```python
from build123d import *

# Parameters (mm, degrees)
SKETCH2_W                = 12
SKETCH2_H                = 90
BOSS_EXTRUDE1_DEPTH      = 10
FILLET1_R                = 5
CUT_EXTRUDE1_DEPTH       = 3
CUT_EXTRUDE2_START       = 7
SKETCH3_2_W              = 12
SKETCH3_2_H              = 9
CUT_EXTRUDE2_DEPTH       = 3
CUT_EXTRUDE4_START       = -4
CUT_EXTRUDE4_DEPTH       = 51.486557197
SKETCH7_R                = 1.5
CUT_EXTRUDE5_DEPTH       = 46.934736311
BOSS_EXTRUDE2_DEPTH      = 7
BOSS_EXTRUDE2_DEPTH_BACK = 7
SKETCH9_W                = 15
SKETCH9_H                = 60
FILLET3_R                = 7


with BuildPart() as part:
    # Sketch2 → Boss-Extrude1 (new body)
    with BuildSketch(Plane.XY):
        Rectangle(SKETCH2_W, SKETCH2_H)
    extrude(amount=BOSS_EXTRUDE1_DEPTH)

    # Fillet1
    fillet1_edges = [part.edges().sort_by_distance(p)[0] for p in [
        (-6, 0, 0),
        (6, 0, 0),
        (6, 0, 10),
        (-6, 0, 10),
    ]]
    fillet(fillet1_edges, radius=FILLET1_R - 0.0001)  # a hair under: the kernel refuses the full size

    # Sketch3 → Cut-Extrude1 (cut)
    with BuildSketch(Plane.XY):
        with BuildLine():
            Line((-6, -36), (-4.5, -40.5))
            ThreePointArc((-4.5, -40.5), (0, -45), (4.5, -40.5))
            Line((4.5, -40.5), (6, -36))
            Line((6, -36), (-6, -36))
        make_face()
        with BuildLine():
            Line((-3.9e-08, -45), (6, -45))
            Line((6, -45), (6, -36))
            Line((6, -36), (4.5, -40.5))
            ThreePointArc((4.5, -40.5), (3.181980501, -43.681980529), (-3.9e-08, -45))
        make_face()
        with BuildLine():
            Line((-6, -45), (-3.9e-08, -45))
            ThreePointArc((-3.9e-08, -45), (-3.181980529, -43.681980501), (-4.5, -40.5))
            Line((-4.5, -40.5), (-6, -36))
            Line((-6, -36), (-6, -45))
        make_face()
    cut_extrude1 = extrude(amount=CUT_EXTRUDE1_DEPTH, mode=Mode.SUBTRACT)

    # Sketch3<2> → Cut-Extrude2 (cut)
    with BuildSketch(Plane.XY.offset(CUT_EXTRUDE2_START)):
        with Locations((0, -40.5)):
            Rectangle(SKETCH3_2_W, SKETCH3_2_H)
    cut_extrude2 = extrude(amount=CUT_EXTRUDE2_DEPTH, mode=Mode.SUBTRACT)

    # Mirror1: Cut-Extrude1, Cut-Extrude2 across plane
    add(cut_extrude1.mirror(Plane.ZX), mode=Mode.SUBTRACT)
    add(cut_extrude2.mirror(Plane.ZX), mode=Mode.SUBTRACT)

    # Sketch3<4> → Cut-Extrude4 (cut)
    with BuildSketch(Plane.XY.offset(CUT_EXTRUDE4_START)):
        with BuildLine():
            Line((-3.9e-08, -45), (6, -45))
            Line((6, -45), (6, -36))
            Line((6, -36), (4.5, -40.5))
            ThreePointArc((4.5, -40.5), (3.181980501, -43.681980529), (-3.9e-08, -45))
        make_face()
        with BuildLine():
            Line((-6, -45), (-3.9e-08, -45))
            ThreePointArc((-3.9e-08, -45), (-3.181980529, -43.681980501), (-4.5, -40.5))
            Line((-4.5, -40.5), (-6, -36))
            Line((-6, -36), (-6, -45))
        make_face()
    cut_extrude4 = extrude(amount=CUT_EXTRUDE4_DEPTH, mode=Mode.SUBTRACT)

    # Sketch7 → Cut-Extrude5 (cut, through all)
    with BuildSketch(Plane(origin=(0, 0, 3), x_dir=(-1, 0, 0), z_dir=(0, 0, -1))):
        with Locations((0, -40.5)):
            Circle(SKETCH7_R)
    cut_extrude5 = extrude(amount=-CUT_EXTRUDE5_DEPTH, mode=Mode.SUBTRACT)

    # Mirror3: Cut-Extrude5 across plane
    add(cut_extrude5.mirror(Plane.ZX), mode=Mode.SUBTRACT)

    # Mirror4: Cut-Extrude4 across plane
    add(cut_extrude4.mirror(Plane.ZX), mode=Mode.SUBTRACT)

    # Sketch9 → Boss-Extrude2 (add, two sides: drawn at the far end of the back side and taken through both)
    with BuildSketch(Plane.XY.offset(5).offset(-BOSS_EXTRUDE2_DEPTH_BACK)):
        Rectangle(SKETCH9_W, SKETCH9_H)
    extrude(amount=BOSS_EXTRUDE2_DEPTH + BOSS_EXTRUDE2_DEPTH_BACK)

    # Fillet3
    fillet3_edges = [part.edges().sort_by_distance(p)[0] for p in [
        (-7.5, 0, 12),
        (7.5, 0, 12),
        (7.5, 0, -2),
        (-7.5, 0, -2),
    ]]
    fillet(fillet3_edges, radius=FILLET3_R - 0.0001)  # a hair under: the kernel refuses the full size


solid = part.part
```
Can you work these out from the model? Positions are in its coordinate system, mm. A direction names the side the tool comes from. Coordinates: 2 decimals unless noted, no trailing zeros. Loops run counter-clockwise (first coordinate to the right, second up) from the corner with the lowest first, then second, coordinate; pieces in that order, holes last.
Item 1: Please list where these lines run through material, in increasing order: L1, parallel to Y at x = 0, z = 4.2; L2, parallel to X at y = 40.5, z = 4.9; L3, parallel to Y at x = -1, z = 6.5.
Answers below:
L1: y = -45 to -42, -39 to 39, 42 to 45
L2: x = -4.5 to -1.5, 1.5 to 4.5
L3: y = -44.89 to -41.62, -39.38 to 39.38, 41.62 to 44.89
Item 2: If we mould it in two halves opening along Y, with no side actions, what happens to faces 1 (the face through (0, 33, 10)), 2 (the face through (5.26, -38.22, 4.97)), 3 (the face through (0, 36, 8)), 4 (the face through (0, -42, 5))? For each: released by +Y, released by -Y, zero draft, split by the parting line, or undercut.
Answers below:
face 1: zero draft
face 2: released by -Y
face 3: released by +Y
face 4: undercut
Item 3: I'm going to push flat-ended pins straight in: pin 1 (2 mm diameter, centred on x = 0.5, y = 32, fed in from -Z); pin 2 (0.9 mm diameter, centred on x = 2.5, z = 2, fed in from +Y); pin 3 (7 mm diameter, centred on x = 0.5, y = 42.5, fed in from +Z); pin 4 (3 mm diameter, centred on y = -1.5, z = 5.5, fed in from -X). Where does each tip first touch, or does it pass through?
Answers below:
pin 1: stops at z = 0
pin 2: stops at y = 36
pin 3: stops at z = 7
pin 4: stops at x = -7.5
Item 4: Suppose I cut it at B-B (z = 8.25). Please give me the cut outline in (x, y).
Answers below:
outline: (-6.7, -30) - (-4.8, -30) - (-4.8, -36) - (4.8, -36) - (4.8, -30) - (6.7, -30) - (6.7, 30) - (4.8, 30) - (4.8, 36) - (-4.8, 36) - (-4.8, 30) - (-6.7, 30) - close
Item 5: Suppose I cut it at C-C (x = 2.5). Please give me the cut outline in (y, z).
Answers below:
outline: (-44.24, 3) - (-36, 3) - (-36, 0.23) - (-30, 0.23) - (-30, -1.71) - (30, -1.71) - (30, 0.23) - (36, 0.23) - (36, 3) - (44.24, 3) - (44.24, 7) - (36, 7) - (36, 9.77) - (30, 9.77) - (30, 11.71) - (-30, 11.71) - (-30, 9.77) - (-36, 9.77) - (-36, 7) - (-44.24, 7) - close
Item 6: Which directions (+Z, -Z, +X, -X, +Y, -Y) give clear straight access to the entire face, cutting with the end or side of a thin tool? Please do faces 5 (the face through (-5, -34, 8)), 6 (the face through (-5, 33, 2)), 7 (the face through (5, -33, 8)).
Answers below:
face 5: +Z, -X, -Y
face 6: -Z, -X, +Y
face 7: +Z, +X, -Y
